Drawing for the job (mm, zero at the part's lowest x, y, z). Give positions to 0.01 mm unless a question says otherwise; leave off trailing zeros. Order: outer loops, then holes, each group sorted by start corner. A loop starts at its lowest first (then second) coordinate and runs counter-clockwise, first axis right, second up. Notation, with made-up numbers: M 60,14.5 L 64,14.5 A23 cw 64,50.5 Z; hole C 28,56 d9. An arc over 180 degrees is marked long. Answer as a JSON object with one key per item and string values.
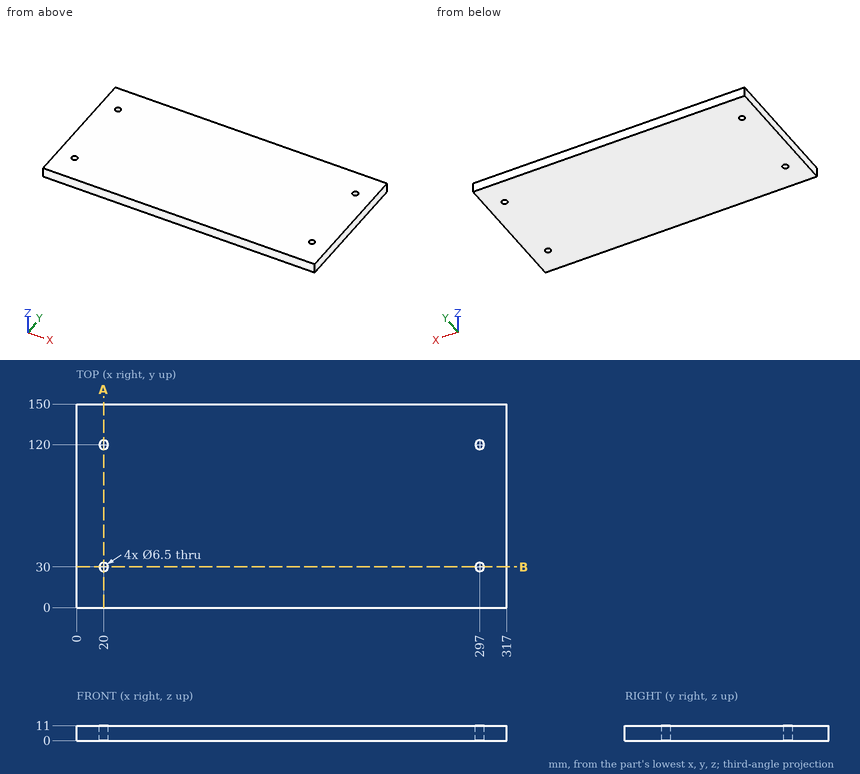
1. Cut at B-B on y = 30. Give the cut face in (x, z), plus the area to 3 significant figures.
Worked answers:
{"outline": "M 0,0 L 16.75,0 L 16.75,11 L 0,11 Z; M 23.25,0 L 293.75,0 L 293.75,11 L 23.25,11 Z; M 300.25,0 L 317,0 L 317,11 L 300.25,11 Z", "area": "3,340 mm^2"}
2. Probe line 1 along Y through (x, z) = (20, 7); line 2 along Y through (x, z) = (21, 1.75); line 3 along X through (y, z) = (28, 6.5). List the from-to ranges inside material, lowest first.
Worked answers:
{"line 1": "y = 0 to 26.75, 33.25 to 116.75, 123.25 to 150", "line 2": "y = 0 to 26.91, 33.09 to 116.91, 123.09 to 150", "line 3": "x = 0 to 17.44, 22.56 to 294.44, 299.56 to 317"}
3. Cut at A-A on x = 20. Give the cut face in (y, z).
Worked answers:
{"outline": "M 0,0 L 26.75,0 L 26.75,11 L 0,11 Z; M 33.25,0 L 116.75,0 L 116.75,11 L 33.25,11 Z; M 123.25,0 L 150,0 L 150,11 L 123.25,11 Z"}
